```python
from build123d import *

# Parameters (mm, degrees)
SKETCH1_W                = 37.5
SKETCH1_H                = 16
BOSS_EXTRUDE1_DEPTH      = 2
SKETCH2_W                = 26
SKETCH2_H                = 14
BOSS_EXTRUDE2_DEPTH      = 1
BOSS_EXTRUDE3_DEPTH      = 2
BOSS_EXTRUDE4_DEPTH      = 6.75
BOSS_EXTRUDE4_DEPTH_BACK = 6.75
CUT_EXTRUDE1_DEPTH       = 27.925824036
CUT_EXTRUDE1_DEPTH_BACK  = 27.925824036
SKETCH5_W                = 2
SKETCH5_H                = 1.5


with BuildPart() as part:
    # Sketch1 → Boss-Extrude1 (new body)
    with BuildSketch(Plane.XY):
        Rectangle(SKETCH1_W, SKETCH1_H)
    extrude(amount=BOSS_EXTRUDE1_DEPTH)

    # Sketch2 → Boss-Extrude2 (add)
    with BuildSketch(Plane.XY.offset(2)):
        with Locations((-5.5, 0)):
            Rectangle(SKETCH2_W, SKETCH2_H)
    extrude(amount=BOSS_EXTRUDE2_DEPTH)

    # Sketch3 → Boss-Extrude3 (add)
    with BuildSketch(Plane.XY.offset(2)):
        Polygon((18.3, -5.25), (18.5, -5.25), (18.5, -7.25), (16.5, -7.25), (16.5, -5.25), (16.7, -5.25), (16.7, -4.75), (16.5, -4.75), (16.5, -2.75), (16.7, -2.75), (16.7, -2.25), (16.5, -2.25), (16.5, -0.25), (16.7, -0.25), (16.7, 0.25), (16.5, 0.25), (16.5, 2.25), (16.7, 2.25), (16.7, 2.75), (16.5, 2.75), (16.5, 4.75), (16.7, 4.75), (16.7, 5.25), (16.5, 5.25), (16.5, 7.25), (18.5, 7.25), (18.5, 5.25), (18.3, 5.25), (18.3, 4.75), (18.5, 4.75), (18.5, 2.75), (18.3, 2.75), (18.3, 2.25), (18.5, 2.25), (18.5, 0.25), (18.3, 0.25), (18.3, -0.25), (18.5, -0.25), (18.5, -2.25), (18.3, -2.25), (18.3, -2.75), (18.5, -2.75), (18.5, -4.75), (18.3, -4.75), align=None)
    extrude(amount=BOSS_EXTRUDE3_DEPTH)

    # Sketch4 → Boss-Extrude4 (add, two sides: drawn at the far end of the back side and taken through both)
    with BuildSketch(Plane(origin=(0, 0, 0), x_dir=(1, 0, 0), z_dir=(0, 1, 0)).offset(-BOSS_EXTRUDE4_DEPTH_BACK)):
        with BuildLine():
            Line((17, -4), (17, -5))
            ThreePointArc((17, -5), (17.292893219, -5.707106781), (18, -6))
            Line((18, -6), (25, -6))
            Line((25, -6), (25, -5))
            Line((25, -5), (18.5, -5))
            ThreePointArc((18.5, -5), (18.146446609, -4.853553391), (18, -4.5))
            Line((18, -4.5), (18, -4))
            Line((18, -4), (17, -4))
        make_face()
    extrude(amount=BOSS_EXTRUDE4_DEPTH + BOSS_EXTRUDE4_DEPTH_BACK)

    # Sketch5 → Cut-Extrude1 (cut, two sides: drawn at the far end of the back side and taken through both)
    with BuildSketch(Plane(origin=(0, 0, 0), x_dir=(0, 0, -1), z_dir=(1, 0, 0)).offset(-CUT_EXTRUDE1_DEPTH_BACK)):
        with Locations((-5, -5)):
            Rectangle(SKETCH5_W, SKETCH5_H)
        with Locations((-5, -2.5)):
            Rectangle(SKETCH5_W, SKETCH5_H)
        with Locations((-5, 0)):
            Rectangle(SKETCH5_W, SKETCH5_H)
        with Locations((-5, 2.5)):
            Rectangle(SKETCH5_W, SKETCH5_H)
        with Locations((-5, 5)):
            Rectangle(SKETCH5_W, SKETCH5_H)
    extrude(amount=CUT_EXTRUDE1_DEPTH + CUT_EXTRUDE1_DEPTH_BACK, mode=Mode.SUBTRACT)


solid = part.part
```
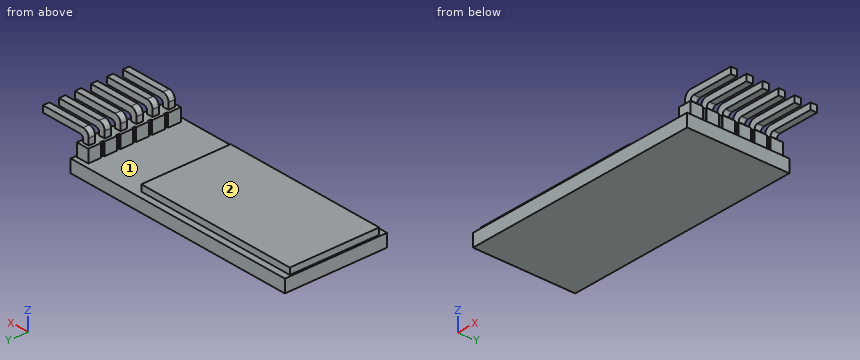
Can you work these out from the model? Positions are in its coordinate system, mm. Face numbers are marked on the shaded views. Coordinates: 2 decimals unless noted, no trailing zeros. Loops run counter-clockwise (first coordinate to the right, second up) from the corner with the lowest first, then second, coordinate; pieces in that order, holes last. Notation, with made-up numbers: (21, 85.25) - (43, 85.25) arc R28 ccw to (43, 106.25) - close; hole circle Ø7 at (-4.75, -34). An arc over 180 degrees is marked (long way). Use a Markdown table: item, result.
Item 1: Will these pins go through, and if not, where does the flat tip stop? pin 1 (0.6 mm diameter, centred on x = 21.5, z = 5.5, fed in from -Y); pin 2 (2 mm diameter, centred on x = -5.5, z = 3.5, fed in from -Y); pin 3 (2 mm diameter, centred on x = 17, z = 3.5, fed in from -Y).
Numbers:
| item | result |
|---|---|
| pin 1 | stops at y = -6.75 |
| pin 2 | stops at y = -7 |
| pin 3 | stops at y = -7.25 |
Item 2: I want a section at D-D on x = 12. Please give me the cut outline in (y, z).
Numbers:
| item | result |
|---|---|
| outline | (-8, 0) - (8, 0) - (8, 2) - (-8, 2) - close |
Item 3: I want a section at B-B on x = -2. Please give me the cut outline in (y, z), and give its area (3 significant figures).
Numbers:
| item | result |
|---|---|
| outline | (-8, 0) - (8, 0) - (8, 2) - (7, 2) - (7, 3) - (-7, 3) - (-7, 2) - (-8, 2) - close |
| area | 46.0 mm2 |
Item 4: I want a section at A-A on x = 21. Please give me the cut outline in (y, z), and give its area (3 significant figures).
Numbers:
| item | result |
|---|---|
| outline | (-6.75, 5) - (-5.75, 5) - (-5.75, 6) - (-6.75, 6) - close; (-4.25, 5) - (-3.25, 5) - (-3.25, 6) - (-4.25, 6) - close; (-1.75, 5) - (-0.75, 5) - (-0.75, 6) - (-1.75, 6) - close; (0.75, 5) - (1.75, 5) - (1.75, 6) - (0.75, 6) - close; (3.25, 5) - (4.25, 5) - (4.25, 6) - (3.25, 6) - close; (5.75, 5) - (6.75, 5) - (6.75, 6) - (5.75, 6) - close |
| area | 6.00 mm2 |
Item 5: If I drill on probe 1 along X at (y, z) = (-4.25, 2.3); probe 2 along X at (y, z) = (5.5, 3.15); probe 3 along Z at (x, y) = (-1, -4), over which ranges is the centre line in solid material (lowest first)? Write a range as from..to.
Numbers:
| item | result |
|---|---|
| probe 1 | x = -18.5..7.5, 16.5..18.5 |
| probe 2 | x = 16.5..18.5 |
| probe 3 | z = 0..3 |
Item 6: I want a section at C-C on z = 1.25. Please give me the cut outline in (x, y), and give its area (3 significant figures).
Numbers:
| item | result |
|---|---|
| outline | (-18.75, -8) - (18.75, -8) - (18.75, 8) - (-18.75, 8) - close |
| area | 600 mm2 |
Item 7: We'd pull the mould along X, two halves only. Please class the marked faces 1 and 2: released by +X, released by -X, zero draft, split by the parting line, or undercut.
Numbers:
| item | result |
|---|---|
| face 1 | undercut |
| face 2 | zero draft |
